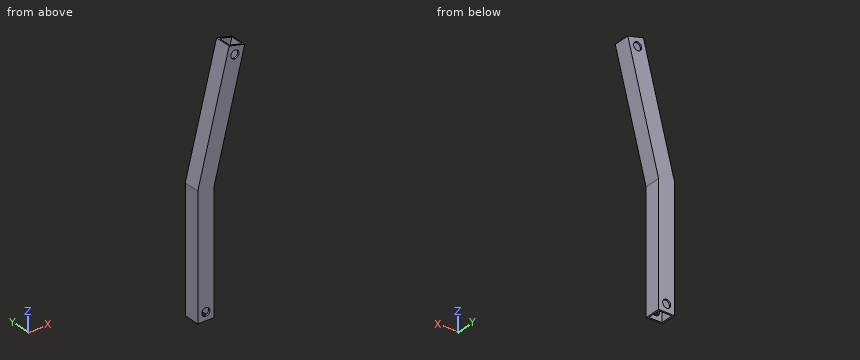
```python
from build123d import *

# Parameters (mm, degrees)
PAD_DEPTH    = 10
THICKNESS_T  = -1
SKETCH001_R  = 2.5
POCKET_DEPTH = 10.001


with BuildPart() as part:
    # Sketch → Pad (new body)
    with BuildSketch(Plane.XZ):
        Polygon((-5, -5), (-5, 70.632568), (14.402741, 146.08767), (24.08767, 143.597259), (5, 69.367432), (5, -5), align=None)
    extrude(amount=PAD_DEPTH)

    # Thickness
    thickness_openings = [part.faces().sort_by_distance(p)[0] for p in [
        (19.245205, -5, 144.842465),
        (0, -5, -5),
    ]]
    offset(amount=THICKNESS_T, openings=thickness_openings)

    # Sketch001 (on Face6 of Thickness) → Pocket (cut, through all)
    with BuildSketch(Plane.XZ.offset(10)):
        with Locations((18, 140)):
            Circle(SKETCH001_R)
        Circle(SKETCH001_R)
    extrude(amount=-POCKET_DEPTH, mode=Mode.SUBTRACT)


solid = part.part
```
The listing builds one solid part. Answer for the finished solid, in the listing's coordinates (mm). Coordinates: 2 decimals unless noted, no trailing zeros. Loops run counter-clockwise (first coordinate to the right, second up) from the corner with the lowest first, then second, coordinate; pieces in that order, holes last. Notation, with made-up numbers: M -18.75,63.5 L -10.75,63.5 A26 cw -10.75,100.5 Z; hole C 11.25,39 d6. An arc over 180 degrees is marked long. Answer as a JSON object with one key per item and string values. Group by question number.
Item 1: Section B-B (z = 46) is taken. Write down the section's boundary in (x, y), and give its area (3 significant figures).
Item 2: Section D-D (z = 0) is taken. Write down the section's boundary in (x, y), and give its area (3 significant figures).
Item 3: Section A-A (y = -6.25) is taken. Write down the section's boundary in (x, z), and give its area (3 significant figures).
Item 4: Section C-C (x = 0) is taken. Write down the section's boundary in (y, z).
Item 5: Consider L1, parallel to X at y = -1.5, z = 53; L2, parallel to Y at x = 2.25, z = 39.5; L3, parallel to X at y = -0.35, z = 140. Determine where each line is inside the solid, lowest interval first.
Item 6: Each of these flat-tipped pins is pushed along its axis until it touches: P1, Ø1.5, axis at y = -4.5, z = 71, coming from the +X side; P2, Ø5, axis at y = -4, z = 117.5, coming from the -X side; P3, Ø1.5, axis at y = -1.5, z = 31.5, coming from the +X side. Where does it stop, or does it pass through?
Solved:
{
 "1": {"outline": "M -5,-10 L 5,-10 L 5,0 L -5,0 Z; hole M -4,-9 L 4,-9 L 4,-1 L -4,-1 Z", "area": "36.0 mm2"},
 "2": {"outline": "M -5,-10 L -2.5,-10 L -2.5,-9 L -4,-9 L -4,-1 L -2.5,-1 L -2.5,0 L -5,0 Z; M 2.5,-10 L 5,-10 L 5,0 L 2.5,0 L 2.5,-1 L 4,-1 L 4,-9 L 2.5,-9 Z", "area": "26.0 mm2"},
 "3": {"outline": "M -5,-5 L -4,-5 L -4,70.51 L 15.37,145.84 L 14.4,146.09 L -5,70.63 Z; M 4,-5 L 5,-5 L 5,69.37 L 24.09,143.6 L 23.12,143.85 L 4.03,69.62 A1 ccw 4,69.37 Z", "area": "305 mm2"},
 "4": {"outline": "M -10,-5 L -9,-5 L -9,-2.5 L -10,-2.5 Z; M -10,2.5 L -9,2.5 L -9,86.06 L -1,86.06 L -1,2.5 L 0,2.5 L 0,90.08 L -10,90.08 Z; M -1,-5 L 0,-5 L 0,-2.5 L -1,-2.5 Z"},
 "5": {"L1": "x = -5 to -4, 4 to 5", "L2": "y = -10 to -9, -1 to 0", "L3": "x = 12.84 to 15.5, 20.5 to 23.16"},
 "6": {"P1": "stops at x = 5.61", "P2": "stops at x = 6.41", "P3": "stops at x = 5"}
}
